Build history of the part. All positions in model axes, mm. Give positions to 0.01 mm unless a question says otherwise; leave off trailing zeros. Loops run counter-clockwise (first coordinate to the right, second up) from the corner with the lowest first, then second, coordinate; pieces in that order, holes last. Notation, with made-up numbers: (69, -8.75) - (96, -8.75) arc R29 ccw to (96, 20.25) - close; hole circle Ø7 at (50, -23). An arc over 180 degrees is marked (long way). Return JSON: item names as keys, results as strings. Group by question number.
1) Mould opens along X. For faces 1 (the face through (-1, 0, -1)), 2 (the face through (-76.8, 0.5, 57.6)) say: released by +X, released by -X, zero draft, split by the parting line, or undercut.
2) Drill centre line: probe 1 along X at (y, z) = (0.4, 60). Where is it in solid material? Low to high. Write a range as from..to.
3) Slice it at B-B (x = 75). List the corners of the cut face in (y, z).
4) Drop a flat-ended pin along its axis: pin 1 (5.5 mm diameter, centred on x = -75, z = 60, fed in from +Y). Give the stop position or say it passes through.
5) Slice it at A-A (z = 60). List the corners of the cut face in (x, y).
```python
from build123d import *

# Parameters (mm, degrees)
IZIM1_W                     = 180
IZIM1_H                     = 150
Y_KSEKLIK_EKSTR_ZYON1_DEPTH = 1
IZIM2_R                     = 3
KES_EKSTR_ZYON1_DEPTH       = 25


with BuildPart() as part:
    # Çizim1 → Yükseklik-Ekstrüzyon1 (new body)
    with BuildSketch(Plane(origin=(0, 0, 0), x_dir=(1, 0, 0), z_dir=(0, 1, 0))):
        Rectangle(IZIM1_W, IZIM1_H)
    extrude(amount=Y_KSEKLIK_EKSTR_ZYON1_DEPTH)

    # Çizim2 → Kes-Ekstrüzyon1 (cut, symmetric)
    with BuildSketch(Plane(origin=(0, 1, 0), x_dir=(1, 0, 0), z_dir=(0, 1, 0))):
        with Locations(Location((-75, 60, 0), (0, 0, 270))):
            Circle(IZIM2_R)
        with Locations(Location((75, 60, 0), (0, 0, 270))):
            Circle(IZIM2_R)
        with Locations(Location((75, -60, 0), (0, 0, 270))):
            Circle(IZIM2_R)
        with Locations(Location((-75, -60, 0), (0, 0, 270))):
            Circle(IZIM2_R)
    extrude(amount=KES_EKSTR_ZYON1_DEPTH, both=True, mode=Mode.SUBTRACT)


solid = part.part
```
Results:
{
 "1": {"face 1": "zero draft", "face 2": "undercut"},
 "2": {"probe 1": "-90..-78, -72..72, 78..90"},
 "3": {"outline": "(0, -75) - (1, -75) - (1, -63) - (0, -63) - close; (0, -57) - (1, -57) - (1, 57) - (0, 57) - close; (0, 63) - (1, 63) - (1, 75) - (0, 75) - close"},
 "4": {"pin 1": "through"},
 "5": {"outline": "(-90, 0) - (-78, 0) - (-78, 1) - (-90, 1) - close; (-72, 0) - (72, 0) - (72, 1) - (-72, 1) - close; (78, 0) - (90, 0) - (90, 1) - (78, 1) - close"}
}
